```python
from build123d import *

# Parameters (mm, degrees)
F1_DEPTH = 76.2
F3_DEPTH = 63.5
F4_R     = 9.525
F5_DEPTH = 101.6


with BuildPart() as f1:
    # F0 (on Front) → F1 (new body)
    with BuildSketch(Plane.XZ):
        Polygon((0, 50.8), (0, 0), (88.9, 0), (38.1, 50.8), align=None)
    extrude(amount=F1_DEPTH)

    # F2 (on face) → F3 (cut)
    with BuildSketch(Plane.XZ.offset(76.2)):
        Polygon((0, 50.8), (0, 44.45), (36.038775, 44.45), (80.102558, 0), (88.9, 0), (38.1, 50.8), align=None)
    extrude(amount=-F3_DEPTH, mode=Mode.SUBTRACT)

    # F4 (on face) → F5 (cut)
    with BuildSketch(Plane(origin=(0, 0, 0), x_dir=(0, -1, 0), z_dir=(-1, 0, 0))):
        with Locations((44.45, 25.4)):
            Circle(F4_R)
    extrude(amount=-F5_DEPTH, mode=Mode.SUBTRACT)


solid = f1.part
```
Model file for the job. Use its own axes, mm. A direction names the side the tool comes from. Coordinates: 2 decimals unless noted, no trailing zeros. Write each loop counter-clockwise with the first axis right and the second up, starting at its lowest first coordinate (ties: lowest second). Pieces come first, ordered by that corner, then holes. Notation, with made-up numbers: (6.25, 24.5) - (38.25, 24.5) arc R23 ccw to (38.25, 54.5) - close; hole circle Ø1 at (-26, -12.75). An arc over 180 degrees is marked (long way). Use a Markdown table: item, result. Add a question column.
Item 1: 3-axis set-ups, long thin cutter, end or side, ignore diameter. For faces 5 (the face through (62.658, -37.839, 17.597)), 6 (the face through (0, -29, 26)), 7 (the face through (18, -45, 44.45)): which of +Z, -Z, +X, -X, +Y, -Y reach the whole face in a straight line?
Item 2: Band-saw the part on A-A, the plane x = 35. Write the cut outline in (y, z) (3 decimals).
Item 3: Two-plate mould, pull along Z, no slides. Class faces 1 (the face through (44, -38, 0)), 2 (the face through (24.7, -42.4, 16.1)), 3 (the face through (19, -6, 50.8)), 4 (the face through (31, -76.2, 18)): pulls with the +Z half, pulls with the -Z half, needs draft (parallel to the pull), parting line crosses it, or undercut.
Item 4: Band-saw the part on B-B, the plane y = -49. Write the cut outline in (x, z), and give its area (3 significant figures).
Item 5: Drop flat-ended pins along their axis: pin 1 (2 mm diameter, centred on x = 45, y = -41, fed in from +Z); pin 2 (8 mm diameter, centred on x = 71, z = 19.5, fed in from -Y); pin 3 (4 mm diameter, centred on x = 27.5, y = -20, fed in from +Z); pin 4 (11.5 mm diameter, centred on y = -44.45, z = 25.4, fed in from +X). Give the stop position or say it passes through.
Item 6: Drill centre lines: line 1 along Y through (x, z) = (33, 25.4) (3 decimals); line 2 along Y through (x, z) = (61, 25.5); line 3 along Z through (x, y) = (37.5, -44.45) (3 decimals). Where is each one in solid material? Low to high.
Item 7: Band-saw the part on D-D, the plane x = 46. Write the cut outline in (y, z) (3 decimals), and give its area (3 significant figures).
Item 8: Band-saw the part on C-C, the plane z = 29. Write the cut outline in (x, y).
A:
| question | item | result |
|---|---|---|
| 1 | face 5 | +Z, +X, -Y |
| 1 | face 6 | +Z, -Z, -X, +Y, -Y |
| 1 | face 7 | +Z, +X, -X, -Y |
| 2 | outline | (-76.2, 0) - (0, 0) - (0, 50.8) - (-12.7, 50.8) - (-12.7, 44.45) - (-76.2, 44.45) - close; hole circle Ø19.05 at (-44.45, 25.4) |
| 3 | face 1 | pulls with the -Z half |
| 3 | face 2 | undercut |
| 3 | face 3 | pulls with the +Z half |
| 3 | face 4 | needs draft |
| 4 | outline | (0, 0) - (80.1, 0) - (63.22, 17.03) - (0, 17.03) - close; (0, 33.77) - (46.63, 33.77) - (36.04, 44.45) - (0, 44.45) - close |
| 4 | area | 1,660 mm² |
| 5 | pin 1 | stops at z = 36.42 |
| 5 | pin 2 | stops at y = -12.7 |
| 5 | pin 3 | stops at z = 44.45 |
| 5 | pin 4 | passes through |
| 6 | line 1 | y = -76.2 to -53.975, -34.925 to 0 |
| 6 | line 2 | y = -12.7 to 0 |
| 6 | line 3 | z = 0 to 15.875, 34.925 to 42.976 |
| 7 | outline | (-76.2, 0) - (0, 0) - (0, 42.9) - (-12.7, 42.9) - (-12.7, 34.401) - (-41.336, 34.401) arc R9.525 cw (long way) to (-47.564, 34.401) - (-76.2, 34.401) - close |
| 7 | area | 2,450 mm² |
| 8 | outline | (0, -76.2) - (51.35, -76.2) - (51.35, -53.27) - (0, -53.27) - close; (0, -35.63) - (51.35, -35.63) - (51.35, -12.7) - (59.9, -12.7) - (59.9, 0) - (0, 0) - close |
